Build history of the part. All positions in model axes, mm. Face numbers are marked on the shaded views. Give positions to 0.01 mm unless a question says otherwise; leave off trailing zeros. Loops run counter-clockwise (first coordinate to the right, second up) from the corner with the lowest first, then second, coordinate; pieces in that order, holes last. Notation, with made-up numbers: (23.5, 53.25) -> (51.5, 53.25) arc R21 ccw to (51.5, 65.25) -> close; hole circle Ø11 at (81, 0). An arc over 180 degrees is marked (long way). Answer as a JSON object with one key per item and string values. Group by question number.
Q1. Band-saw the part on C-C, the plane x = 265.5. Write the cut outline in (y, z), plus the area to 3 significant figures.
Q2. Band-saw the part on B-B, the plane z = -119. Write the cut outline in (x, y).
Q3. Two-plate mould, pull along X, no slides. Class the marked faces 1, 2 and 3: pulls with the +X half, pulls with the -X half, needs draft (parallel to the pull), parting line crosses it, or undercut.
Q4. Band-saw the part on A-A, the plane y = -55. Write the cut outline in (x, z), plus the area to 3 significant figures.
Q5. Wall check: probe 1 along X at (y, z) = (-8, -93); probe 2 along Z at (x, y) = (368, -4); probe 3 along X at (y, z) = (-75.5, -99). Give the ranges that are in metal, low to high. Write a range as from..to.
Q6. Drop flat-ended pins along their axis: pin 1 (12.5 mm diameter, centred on x = 458.5, y = -59, fed in from -Z); pin 2 (19 mm diameter, centred on x = 368.1, z = -93.3, fed in from -Y); pin 3 (12.5 mm diameter, centred on x = 49, y = -57.5, fed in from +Z). Give the stop position or say it passes through.
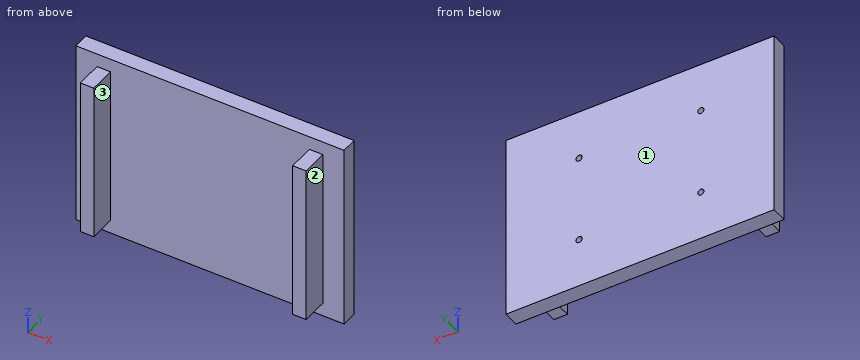
Autodesk Inventor part; units mm, degrees
ref_plane "YZ Plane" through (0, 0, 0) normal (1, 0, 0) x (0, 1, 0)
ref_plane "XZ Plane" through (0, 0, 0) normal (0, 1, 0) x (-1, 0, 0)
ref_plane "XY Plane" through (0, 0, 0) normal (0, 0, 1) x (1, 0, 0)
sketch "Sketch1" plane through (0, 0, 0) normal (0, 1, 0) x (-1, 0, 0)
  line L0 (0, 0) -> (-506.2, 0)
  line L1 (-506.2, 0) -> (-506.2, -351.6)
  line L2 (-506.2, -351.6) -> (0, -351.6)
  line L3 (0, -351.6) -> (0, 0)
  dimension "d0" = 506.2
  dimension "d1" = 351.6
extrude "Extrusion1" add sketch "Sketch1" against normal blind 30
sketch "Sketch2" plane through (0, -30, 0) normal (0, -1, 0) x (1, 0, 0)
  line L0 (466.2, -326.2) -> (440.8, -326.2)
  line L1 (440.8, -326.2) -> (440.8, -25.4)
  line L2 (440.8, -25.4) -> (466.2, -25.4)
  line L3 (466.2, -25.4) -> (466.2, -326.2)
  line L4 (65.4, -326.2) -> (40, -326.2)
  line L5 (40, -326.2) -> (40, -25.4)
  line L6 (40, -25.4) -> (65.4, -25.4)
  line L7 (65.4, -25.4) -> (65.4, -326.2)
  line L8 (506.2, 0) -> (0, 0)
  line L9 (0, -351.6) -> (506.2, -351.6)
  line L10 (0, 0) -> (0, -351.6)
  dimension "d4" = 25.4
  dimension "d5" = 25.4
  dimension "d6" = 25.4
  dimension "d7" = 25.4
  dimension "d9" = 25.4
  dimension "d10" = 25.4
  dimension "d11" = 40
  dimension "d12" = 375.4
extrude "Extrusion2" add sketch "Sketch2" along normal blind 50
sketch "Sketch4" plane through (0, 0, 0) normal (0, 1, 0) x (1, 0, 0)
  line L0 (0, 351.6) -> (0, 0)
  line L1 (506.2, 351.6) -> (0, 351.6)
  line L2 (506.2, 0) -> (506.2, 351.6)
  point P0 (138.1, 258.3)
  point P1 (368.1, 258.3)
  point P2 (138.1, 93.3)
  point P3 (368.1, 93.3)
  dimension "d22" = 230
  dimension "d23" = 230
  dimension "d24" = 165
  dimension "d25" = 165
  dimension "d26" = 138.1
  dimension "d27" = 138.1
  dimension "d28" = 93.3
  dimension "d36" = 93.3
hole "Hole1" at (138.1, 0, -258.3) at (368.1, 0, -258.3) at (138.1, 0, -93.3) at (368.1, 0, -93.3) direction (0, -1, 0) diameter 11.835 depth 12 tip angle 137
equation "\"d6\" = d4"
equation "\"d10\" = d9"
properties part number "Soporte de matriz"
Worked answers:
{
 "1": {"outline": "(-30, -351.6) -> (0, -351.6) -> (0, 0) -> (-30, 0) -> close", "area": "10,500 mm2"},
 "2": {"outline": "(0, -30) -> (40, -30) -> (40, -80) -> (65.4, -80) -> (65.4, -30) -> (440.8, -30) -> (440.8, -80) -> (466.2, -80) -> (466.2, -30) -> (506.2, -30) -> (506.2, 0) -> (0, 0) -> close"},
 "3": {"face 1": "needs draft", "face 2": "pulls with the +X half", "face 3": "undercut"},
 "4": {"outline": "(40, -326.2) -> (65.4, -326.2) -> (65.4, -25.4) -> (40, -25.4) -> close; (440.8, -326.2) -> (466.2, -326.2) -> (466.2, -25.4) -> (440.8, -25.4) -> close", "area": "15,300 mm2"},
 "5": {"probe 1": "0..132.19, 144.01..362.19, 374.01..506.2", "probe 2": "-351.6..-264.22, -252.38..-99.22, -87.38..0", "probe 3": "40..65.4, 440.8..466.2"},
 "6": {"pin 1": "z = -326.2", "pin 2": "y = -30", "pin 3": "z = -25.4"}
}
